Work out the finished part from the listing and answer in its coordinate system (mm). A direction names the side the tool comes from. Give positions to 0.01 mm unless a question says otherwise; leave off trailing zeros. Loops run counter-clockwise (first coordinate to the right, second up) from the corner with the lowest first, then second, coordinate; pieces in that order, holes last.
```python
from build123d import *

# Parameters (mm, degrees)
F0_W     = 120
F0_H     = 95
F1_DEPTH = 10
F2_W     = 115
F2_H     = 90
F3_DEPTH = 7.5
F4_W     = 103
F4_H     = 78
F5_DEPTH = 2.501
F6_R     = 2
F7_R     = 1


with BuildPart() as f1:
    # F0 (on Front) → F1 (new body)
    with BuildSketch(Plane.XZ):
        Rectangle(F0_W, F0_H)
    extrude(amount=F1_DEPTH)

    # F2 (on face) → F3 (cut)
    with BuildSketch(Plane.XZ.offset(10)):
        Rectangle(F2_W, F2_H)
    extrude(amount=-F3_DEPTH, mode=Mode.SUBTRACT)

    # F4 (on face) → F5 (cut, through all)
    with BuildSketch(Plane.XZ.offset(2.5)):
        Rectangle(F4_W, F4_H)
    extrude(amount=-F5_DEPTH, mode=Mode.SUBTRACT)

    # F6
    f6_edges = [f1.edges().sort_by_distance(p)[0] for p in [
        (60, -5, 47.5),
        (60, -5, -47.5),
        (-60, -5, -47.5),
        (-60, -5, 47.5),
    ]]
    fillet(f6_edges, radius=F6_R)

    # F7
    f7_edges = [f1.edges().sort_by_distance(p)[0] for p in [
        (0, 0, 47.5),
        (59.414214, 0, 46.914214),
        (-59.414214, 0, 46.914214),
        (60, 0, 0),
        (-60, 0, 0),
        (59.414214, 0, -46.914214),
        (-59.414214, 0, -46.914214),
        (0, 0, -47.5),
        (0, 0, 39),
        (-51.5, 0, 0),
        (0, 0, -39),
        (51.5, 0, 0),
    ]]
    fillet(f7_edges, radius=F7_R)


solid = f1.part
```
Q1. Section B-B on x = 11.5 is taken. Give the vertices of the cut face in (y, z).
Q2. Consider line 1 along Z through (x, y) = (-42, -5.5); line 2 along X through (y, z) = (-3, -37); line 3 along X through (y, z) = (-1.5, 33.5). Determine where each line is inside the solid, lowest interval first.
Q3. Section C-C on z = 22 is taken. Give the vertices of the cut face in (x, y).
Q4. Section A-A on y = -8 is taken. Give the vertices of the cut face in (x, z), plus the area to 3 significant figures.
Q5. Determine the mould class of faces 1 (the face through (-60, -5, -1)), 2 (the face through (-1, -6, -45)), 3 (the face through (-58, -10, 0)) for opening direction X: +X half, -X half, draft (parallel to the pull), parting line (faces both ways), or undercut.
Q6. Which of the six approach directions +Z, -Z, +X, -X, +Y, -Y give full straight-line access (tool end or side, diameter ignored) to faces 4 (the face through (60, -5, -1)), 5 (the face through (-1, -6, 45))?
Q7. Given pin 1 (8 mm diameter, centred on x = -47, z = -0.5, fed in from +Y), flat-ended and moving along its own axis, determine where the tip first touches the part or whether it passes through.
Check result:
1. outline: (-10, -47.5) - (-1, -47.5) arc R1 ccw to (0, -46.5) - (0, -40) arc R1 ccw to (-1, -39) - (-2.5, -39) - (-2.5, -45) - (-10, -45) - close; (-10, 45) - (-2.5, 45) - (-2.5, 39) - (-1, 39) arc R1 ccw to (0, 40) - (0, 46.5) arc R1 ccw to (-1, 47.5) - (-10, 47.5) - close
2. line 1: z = -47.5 to -45, 45 to 47.5
2. line 2: x = -60 to -57.5, 57.5 to 60
2. line 3: x = -60 to -51.5, 51.5 to 60
3. outline: (-60, -10) - (-57.5, -10) - (-57.5, -2.5) - (-51.5, -2.5) - (-51.5, -1) arc R1 ccw to (-52.5, 0) - (-59, 0) arc R1 ccw to (-60, -1) - close; (51.5, -2.5) - (57.5, -2.5) - (57.5, -10) - (60, -10) - (60, -1) arc R1 ccw to (59, 0) - (52.5, 0) arc R1 ccw to (51.5, -1) - close
4. outline: (-60, -45.5) arc R2 ccw to (-58, -47.5) - (58, -47.5) arc R2 ccw to (60, -45.5) - (60, 45.5) arc R2 ccw to (58, 47.5) - (-58, 47.5) arc R2 ccw to (-60, 45.5) - close; hole (-57.5, -45) - (57.5, -45) - (57.5, 45) - (-57.5, 45) - close
4. area: 1,050 mm2
5. face 1: -X half
5. face 2: undercut
5. face 3: draft
6. face 4: +Z, -Z, +X, +Y, -Y
6. face 5: -Y
7. pin 1: passes through
